Verification items for the finished model (mm, model axes). Coordinates: 2 decimals unless noted, no trailing zeros. Loops run counter-clockwise (first coordinate to the right, second up) from the corner with the lowest first, then second, coordinate; pieces in that order, holes last.
Q1. Sectioned sample at B-B (y = 0). Enter the section's corners in (x, z), then the cut area to 3 significant figures.
Q2. Sectioned sample at A-A (z = 3.5). Enter the section's corners in (x, y), then the cut area to 3 significant figures.
Q3. Material ranges on probe 1 along Y at (x, z) = (0.8, 3.5); probe 2 along Z at (x, y) = (0.85, -1); probe 3 along Y at (x, z) = (1.25, -0.25), recorded low to high.
Q4. Sectioned sample at C-C (x = 1.3). Enter the section's corners in (y, z).
Q5. Go/stop test with a flat-tipped pin: P1, Ø1, axis at x = 0.5, y = -1, coming from the +Z side. Record where the tip stops, or that it passes through.
```python
from build123d import *

# Parameters (mm, degrees)
SKETCH1_R           = 1
SKETCH1_R_2         = 1.25
BOSS_EXTRUDE1_DEPTH = 2


with BuildPart() as part:
    # Sketch1 → Boss-Extrude1 (new body)
    with BuildSketch(Plane(origin=(0, 0, 0), x_dir=(0, 0, -1), z_dir=(1, 0, 0))):
        with BuildLine():
            ThreePointArc((-1.414213562, 4.242640687), (-4.242640687, 4.242640687), (-4.242640687, 1.414213562))
            Line((-4.242640687, 1.414213562), (1.414213562, -4.242640687))
            ThreePointArc((1.414213562, -4.242640687), (4.242640687, -4.242640687), (4.242640687, -1.414213562))
            Line((4.242640687, -1.414213562), (-1.414213562, 4.242640687))
        make_face()
        with Locations((2.828427125, -2.828427125)):
            Circle(SKETCH1_R, mode=Mode.SUBTRACT)
        with Locations((-2.828427125, 2.828427125)):
            Circle(SKETCH1_R, mode=Mode.SUBTRACT)
        Circle(SKETCH1_R_2, mode=Mode.SUBTRACT)
    extrude(amount=BOSS_EXTRUDE1_DEPTH)


solid = part.part
```
Geometry check:
1. outline: (0, -2.83) - (2, -2.83) - (2, -1.25) - (0, -1.25) - close; (0, 1.25) - (2, 1.25) - (2, 2.83) - (0, 2.83) - close
1. area: 6.31 mm2
2. outline: (0, 0.67) - (2, 0.67) - (2, 2.09) - (0, 2.09) - close; (0, 3.57) - (2, 3.57) - (2, 4.71) - (0, 4.71) - close
2. area: 5.12 mm2
3. probe 1: y = 0.67 to 2.09, 3.57 to 4.71
3. probe 2: z = -3.83 to -0.75, 0.75 to 1.83
3. probe 3: y = -3.08 to -1.22, 1.22 to 2.58
4. outline: (-4.24, -1.41) arc R2 ccw to (-1.41, -4.24) - (4.24, 1.41) arc R2 ccw to (1.41, 4.24) - close; hole circle Ø2 at (-2.83, -2.83); hole circle Ø2.5 at (0, 0); hole circle Ø2 at (2.83, 2.83)
5. P1: stops at z = 2.33
